```python
from build123d import *

# Parameters (mm, degrees)
SKETCH1_W           = 8.5
SKETCH1_H           = 12
SKETCH1_R           = 0.5
SKETCH1_W_2         = 3
SKETCH1_H_2         = 6
BOSS_EXTRUDE1_DEPTH = 1.5
FILLET1_R           = 3


with BuildPart() as part:
    # Sketch1 → Boss-Extrude1 (new body, symmetric)
    with BuildSketch(Plane(origin=(0, 0, 0), x_dir=(1, 0, 0), z_dir=(0, 1, 0))):
        Rectangle(SKETCH1_W, SKETCH1_H)
        with Locations((2.75, 2)):
            Circle(SKETCH1_R, mode=Mode.SUBTRACT)
        with Locations((2.75, -2)):
            Circle(SKETCH1_R, mode=Mode.SUBTRACT)
        with Locations((-0.75, 0)):
            Rectangle(SKETCH1_W_2, SKETCH1_H_2, mode=Mode.SUBTRACT)
    extrude(amount=BOSS_EXTRUDE1_DEPTH, both=True)

    # Fillet1
    fillet1_edges = [part.edges().sort_by_distance(p)[0] for p in [
        (-4.25, 0, -6),
        (4.25, 0, -6),
        (4.25, 0, 6),
        (-4.25, 0, 6),
    ]]
    fillet(fillet1_edges, radius=FILLET1_R)


solid = part.part
```
Input: part model. Units: mm. Frame: model coordinates. A direction names the side the tool comes from. Round coordinates to 2 decimals unless told otherwise and drop trailing zeros. Order: outer loops, then holes, each group sorted by start corner. A loop starts at its lowest first (then second) coordinate and runs counter-clockwise, first axis right, second up. Notation, with made-up numbers: (77.25, -35) - (93.25, -35) arc R27 cw to (93.25, -17) - close; hole circle Ø9 at (69.25, 6). An arc over 180 degrees is marked (long way). Answer in a Markdown table with one row per item.
Item 1: Mould query, pull axis X, two halves, no side actions, for faces 3 (the flat face through (-1, 0, 3)), 4 (the cylindrical face through (-3.39, 0.02, 5.1)), 5 (the flat face through (1, -1.5, 0)). Classes: released by +X, released by -X, zero draft, split by the parting line, or undercut.
Model answer:
| item | result |
|---|---|
| face 3 | undercut |
| face 4 | released by -X |
| face 5 | zero draft |
Item 2: Reachability of faces 1 (the flat face through (0, 0, 6)), 2 (the flat face through (0.75, 0, 0)) from +Z, -Z, +X, -X, +Y, -Y: full face, straight path, thin tool, end or side. Return the list, or none.
Model answer:
| item | result |
|---|---|
| face 1 | +Z, +X, -X, +Y, -Y |
| face 2 | +Y, -Y |
Item 3: Section query C-C (y = 0.25). Return the cut outline in (x, z), then the cut area to 3 significant figures.
Model answer:
| item | result |
|---|---|
| outline | (-4.25, -3) arc R3 ccw to (-1.25, -6) - (1.25, -6) arc R3 ccw to (4.25, -3) - (4.25, 3) arc R3 ccw to (1.25, 6) - (-1.25, 6) arc R3 ccw to (-4.25, 3) - close; hole (-2.25, -3) - (0.75, -3) - (0.75, 3) - (-2.25, 3) - close; hole circle Ø1 at (2.75, -2); hole circle Ø1 at (2.75, 2) |
| area | 74.7 mm² |
Item 4: Section query B-B (z = 2). Return the cut outline in (x, y), then the cut area to 3 significant figures.
Model answer:
| item | result |
|---|---|
| outline | (-4.25, -1.5) - (-2.25, -1.5) - (-2.25, 1.5) - (-4.25, 1.5) - close; (0.75, -1.5) - (2.25, -1.5) - (2.25, 1.5) - (0.75, 1.5) - close; (3.25, -1.5) - (4.25, -1.5) - (4.25, 1.5) - (3.25, 1.5) - close |
| area | 13.5 mm² |
Item 5: Section query D-D (x = 2.75). Return the cut outline in (y, z), then the cut area to 3 significant figures.
Model answer:
| item | result |
|---|---|
| outline | (-1.5, -5.6) - (1.5, -5.6) - (1.5, -2.5) - (-1.5, -2.5) - close; (-1.5, -1.5) - (1.5, -1.5) - (1.5, 1.5) - (-1.5, 1.5) - close; (-1.5, 2.5) - (1.5, 2.5) - (1.5, 5.6) - (-1.5, 5.6) - close |
| area | 27.6 mm² |
Item 6: Section query A-A (x = -1). Return the cut outline in (y, z).
Model answer:
| item | result |
|---|---|
| outline | (-1.5, -6) - (1.5, -6) - (1.5, -3) - (-1.5, -3) - close; (-1.5, 3) - (1.5, 3) - (1.5, 6) - (-1.5, 6) - close |
Item 7: Line query: line 1 (X direction, y = -0.1, z = -2); line 2 (Z direction, x = -0.5, y = 1.15); line 3 (Z direction, x = 2.75, y = 0.05). Output: solid intervals per line, ascending.
Model answer:
| item | result |
|---|---|
| line 1 | x = -4.25 to -2.25, 0.75 to 2.25, 3.25 to 4.25 |
| line 2 | z = -6 to -3, 3 to 6 |
| line 3 | z = -5.6 to -2.5, -1.5 to 1.5, 2.5 to 5.6 |
